Check sheet for the modelled part. Datum: model origin and axes. Units: mm. A direction names the side the tool comes from. Give positions to 0.01 mm unless a question says otherwise; leave off trailing zeros. Order: outer loops, then holes, each group sorted by start corner. A loop starts at its lowest first (then second) coordinate and runs counter-clockwise, first axis right, second up. Notation, with made-up numbers: M 2.25,75 L 7.25,75 A6 ccw 7.25,85 Z; hole C 6.25,27 d3. An arc over 180 degrees is marked long. Return JSON: item names as keys, results as strings. Group by question number.
from build123d import *

# Parameters (mm, degrees)
F1_DEPTH = 12
F2_DEPTH = 50
F3_W     = 56
F3_H     = 34
F4_DEPTH = 25
F5_W     = 50
F5_H     = 20
F6_DEPTH = 25
F8_DEPTH = 4


with BuildPart() as f1:
    # F0 (on Top) → F1 (new body)
    with BuildSketch(Plane.XY):
        Polygon((-27.3359761563, -54), (44.6640238437, -54), (44.6640238437, -50), (44.6640238437, 0), (-39.9199636387, 112.655294226), (-85.9636434561, 78.0847215416), (-27.3359761563, 0), (-27.3359761563, -50), align=None)
        Polygon((39.6640238437, -50.3684133291), (-22.3359761563, -50.1054301858), (-22.3359761563, 0), (-79.7640645644, 76.4870324634), (-40.1153402772, 106.2561367194), (39.6640238437, 0), align=None, mode=Mode.SUBTRACT)
        Polygon((-22.3359761563, 0), (-22.3359761563, -50.1054301858), (39.6640238437, -50.3684133291), (39.6640238437, 0), (-40.1153402772, 106.2561367194), (-79.7640645644, 76.4870324634), align=None)
    extrude(amount=F1_DEPTH)

    # F0 (on Top) → F2 (join)
    with BuildSketch(Plane.XY):
        Polygon((-27.3359761563, -54), (44.6640238437, -54), (44.6640238437, -50), (44.6640238437, 0), (-39.9199636387, 112.655294226), (-85.9636434561, 78.0847215416), (-27.3359761563, 0), (-27.3359761563, -50), align=None)
        Polygon((39.6640238437, -50.3684133291), (-22.3359761563, -50.1054301858), (-22.3359761563, 0), (-79.7640645644, 76.4870324634), (-40.1153402772, 106.2561367194), (39.6640238437, 0), align=None, mode=Mode.SUBTRACT)
    extrude(amount=F2_DEPTH)

    # F3 (on face) → F4 (cut)
    with BuildSketch(Plane.XZ.offset(54)):
        with Locations((8.6640238437, 25)):
            Rectangle(F3_W, F3_H)
    extrude(amount=-F4_DEPTH, mode=Mode.SUBTRACT)

    # F5 (on face) → F6 (cut)
    with BuildSketch(Plane(origin=(-68.4824082667, 91.210004189, 0), x_dir=(-0.7996846585, -0.6004202253, 0), z_dir=(-0.6004202253, 0.7996846585, 0))):
        with Locations((-6.8476465531, 25)):
            Rectangle(F5_W, F5_H)
    extrude(amount=-F6_DEPTH, mode=Mode.SUBTRACT)

    # F7 (on face) → F8 (cut)
    with BuildSketch(Plane.XY.offset(12)):
        Polygon((-49.5763184557, 82.8963528815), (-54.6922828798, 79.0551781388), (4.6640238437, 0), (4.6640238437, -29), (12.6640238437, -29), (12.6640238437, 0), align=None)
    extrude(amount=-F8_DEPTH, mode=Mode.SUBTRACT)


solid = f1.part
1) Sectioned sample at D-D on z = 10. Record the boundary of the cut face in (x, y), then the cut area to 3 significant figures.
2) Tool access check on faces 4 (the face through (-19.336, -52, 19)), 5 (the face through (4.664, -14, 10)), 6 (the face through (-18.02, 40.87, 10.03)). Record the directions out of +Z, -Z, +X, -X, +Y, -Y that give a thin tool (end or side, any length) a straight path to the whole face; none if there is none.
3) Material ranges on line 1 along X through (y, z) = (-45.5, 15.5); line 2 along X through (y, z) = (7, 12.5); line 3 along Z through (x, y) = (-50, 55), recorded low to high.
4) Sectioned sample at B-B on y = -38. Record the boundary of the cut face in (x, z), then the cut area to 3 significant figures.
5) Sectioned sample at C-C on z = 31. Record the boundary of the cut face in (x, y), then the cut area to 3 significant figures.
6) Release check for a two-part mould opening along Z. For faces 1 (the face through (-16, 23, 12)), 2 (the face through (24, -29, 10)), 3 (the face through (8, -52, 42)) record: released by +Z, released by -Z, zero draft, split by the parting line, or undercut.
7) Sectioned sample at A-A on x = 26. Record the boundary of the cut face in (y, z).
8) Depth check by flat-ended pin: P1, Ø15, axis at y = -16, z = 26, coming from the -X side; P2, Ø1, axis at x = -15.5, z = 32, coming from the +Y side; P3, Ø4, axis at y = 10.5, z = 14.5, coming from the -X side. Enter the tip coordinate at first touch or a pass-through.
Reply:
{
 "1": {"outline": "M -85.96,78.08 L -27.34,0 L -27.34,-54 L -19.34,-54 L -19.34,-29 L 4.66,-29 L 4.66,0 L -54.69,79.06 L -49.58,82.9 L 12.66,0 L 12.66,-29 L 36.66,-29 L 36.66,-54 L 44.66,-54 L 44.66,0 L -39.92,112.66 Z", "area": "8,470 mm^2"},
 "2": {"face 4": "-Y", "face 5": "+Z, -Y", "face 6": "+Z"},
 "3": {"line 1": "-27.34 to -22.34, 39.66 to 44.66", "line 2": "-32.59 to -27.59, 34.41 to 39.41", "line 3": "0 to 12"},
 "4": {"outline": "M -27.34,0 L 44.66,0 L 44.66,50 L 39.66,50 L 39.66,12 L 36.66,12 L 36.66,8 L -19.34,8 L -19.34,12 L -22.34,12 L -22.34,50 L -27.34,50 Z", "area": "1,020 mm^2"},
 "5": {"outline": "M -85.96,78.08 L -27.34,0 L -27.34,-54 L -19.34,-54 L -19.34,-50.12 L -22.34,-50.11 L -22.34,0 L -67.76,60.49 L -67.99,60.32 L -83,80.31 Z; M -43.01,110.33 L -28,90.34 L -28.11,90.26 L 39.66,0 L 39.66,-50.37 L 36.66,-50.36 L 36.66,-54 L 44.66,-54 L 44.66,0 L -39.92,112.66 Z", "area": "1,510 mm^2"},
 "6": {"face 1": "released by +Z", "face 2": "zero draft", "face 3": "undercut"},
 "7": {"outline": "M -54,0 L 24.86,0 L 24.86,50 L 18.2,50 L 18.2,12 L -29,12 L -29,8 L -54,8 Z; M -54,42 L -50.31,42 L -50.31,50 L -54,50 Z"},
 "8": {"P1": "x = -27.34", "P2": "y = 80.8", "P3": "x = -36.72"}
}
